from build123d import *

# Parameters (mm, degrees)
BOSS_EXTRUDE1_DEPTH = 1.59
SKETCH2_R           = 1.59
SKETCH2_R_2         = 0.51
CUT_EXTRUDE1_DEPTH  = 68.193958806


with BuildPart() as part:
    # Sketch1 → Boss-Extrude1 (new body)
    with BuildSketch(Plane(origin=(0, 0, 0), x_dir=(1, 0, 0), z_dir=(0, 1, 0))):
        Polygon((-47.5, -36.5), (-36.5, -47.5), (47, -47.5), (47, -40.5), (47.5, -40.5), (47.5, 36.5), (36.5, 47.5), (-47, 47.5), (-47, 40.5), (-47.5, 40.5), align=None)
    extrude(amount=BOSS_EXTRUDE1_DEPTH)

    # Sketch2 → Cut-Extrude1 (cut, through all)
    with BuildSketch(Plane(origin=(0, 1.59, 0), x_dir=(1, 0, 0), z_dir=(0, 1, 0))):
        with Locations(Location((-39.5, -39.5, 0), (0, 0, 270))):
            Circle(SKETCH2_R)
        with Locations(Location((-39.5, 39.5, 0), (0, 0, 270))):
            Circle(SKETCH2_R)
        with Locations(Location((39.5, 39.5, 0), (0, 0, 270))):
            Circle(SKETCH2_R)
        with Locations(Location((39.5, -39.5, 0), (0, 0, 270))):
            Circle(SKETCH2_R)
        with Locations(Location((-2.67, -21.93, 0), (0, 0, 270))):
            Circle(SKETCH2_R_2)
        with Locations(Location((2.03, -22.75, 0), (0, 0, 270))):
            Circle(SKETCH2_R_2)
        with Locations(Location((-2.67, -42.07, 0), (0, 0, 270))):
            Circle(SKETCH2_R_2)
        with Locations(Location((2.03, -41.24, 0), (0, 0, 270))):
            Circle(SKETCH2_R_2)
    extrude(amount=-CUT_EXTRUDE1_DEPTH, mode=Mode.SUBTRACT)


solid = part.part
For this review, take the finished solid that the model builds, in its own axes (mm). Coordinates: 2 decimals unless noted, no trailing zeros. Order: outer loops, then holes, each group sorted by start corner. A loop starts at its lowest first (then second) coordinate and runs counter-clockwise, first axis right, second up. Notation, with made-up numbers: (25.5, -4.5) - (45.5, -4.5) arc R26 cw to (45.5, 9.5) - close; hole circle Ø4 at (28, 60). An arc over 180 degrees is marked (long way). Answer as CSV lines item,"result". Start each with the question number.
1) Add section A-A (x = 39.5). State the section outline as (y, z) points, then the cut area to 3 significant figures.
2) To check wall thickness, follow line 1 along X through (y, z) = (0.95, -39.5); line 2 along X through (y, z) = (1.15, 42.07); line 3 along X through (y, z) = (0.65, 39.5). State the ranges of each line that lie inside material, in increasing order. Write a range as [from, to].
3) Add section B-B (y = 0.5). Count the separate pieces of the cut face and the enclosed holes in it, then the cut area to 3 significant figures.
4) Insertion check: P1, Ø0.8, axis at y = 1, z = -45, coming from the -X side; P2, Ø0.8, axis at x = 2.03, z = 22.75, coming from the -Y side. Each pin has a flat end and moves straight along its axis. Give the tip position at first contact, or say it passes through.
5) Draft analysis for pull direction X (two halves, no side actions). For faces 1 (the flat face through (-1, 1.59, -1)), 2 (the cylindrical face through (39.978, 0.806, 41.017)), 3 (the flat face through (-42, 1, 42)), 4 (the cylindrical face through (-39.022, 0.806, -37.983)), state which applies: +X half, -X half, draft (parallel to the pull), parting line (faces both ways), or undercut.
Result:
1,outline,"(0, -44.5) - (1.59, -44.5) - (1.59, -41.09) - (0, -41.09) - close; (0, -37.91) - (1.59, -37.91) - (1.59, 37.91) - (0, 37.91) - close; (0, 41.09) - (1.59, 41.09) - (1.59, 47.5) - (0, 47.5) - close"
1,area,"136 mm^2"
2,line 1,"[-47.5, -41.09], [-37.91, 37.91], [41.09, 44.5]"
2,line 2,"[-41.93, -3.18], [-2.16, 47]"
2,line 3,"[-44.5, -41.09], [-37.91, 37.91], [41.09, 47.5]"
3,separate pieces,"1"
3,enclosed holes,"8"
3,area,"8,860 mm^2"
4,P1,"x = -47"
4,P2,"through"
5,face 1,"draft"
5,face 2,"undercut"
5,face 3,"-X half"
5,face 4,"undercut"
